```python
from build123d import *

# Parameters (mm, degrees)
SKETCH1_R            = 10
BOSS_EXTRUDE1_DEPTH  = 30
SKETCH2_R            = 12.5
BOSS_EXTRUDE5_DEPTH  = 60
SKETCH5_R            = 14
BOSS_EXTRUDE8_DEPTH  = 70
SKETCH7_R            = 16
BOSS_EXTRUDE9_DEPTH  = 76
SKETCH8_R            = 14
BOSS_EXTRUDE13_DEPTH = 24
SKETCH12_R           = 12.5
BOSS_EXTRUDE15_DEPTH = 150
SKETCH14_R           = 11.5
BOSS_EXTRUDE16_DEPTH = 70
SKETCH15_R           = 10
BOSS_EXTRUDE17_DEPTH = 20
CUT_EXTRUDE1_DEPTH   = 6
CUT_EXTRUDE2_DEPTH   = 8
SKETCH18_R           = 14
CUT_EXTRUDE3_DEPTH   = 264
SKETCH19_R           = 14
BOSS_EXTRUDE18_DEPTH = 45
SKETCH20_R           = 12.5
BOSS_EXTRUDE19_DEPTH = 139
SKETCH21_R           = 11.5
BOSS_EXTRUDE20_DEPTH = 60
SKETCH22_R           = 10
BOSS_EXTRUDE21_DEPTH = 20
CUT_EXTRUDE4_DEPTH   = 8
CUT_EXTRUDE5_DEPTH   = 8
SKETCH26_W           = 1.2
SKETCH26_H           = 1.8
SKETCH30_W           = 1.2
SKETCH30_H           = 1.8
SKETCH31_W           = 1.2
SKETCH31_H           = 1.8
SKETCH34_W           = 1.2
SKETCH34_H           = 1.8
SKETCH35_R           = 14
BOSS_EXTRUDE22_DEPTH = 56
SKETCH36_W           = 1.2
SKETCH36_H           = 1.8


with BuildPart() as part:
    # Sketch1 → Boss-Extrude1 (new body)
    with BuildSketch(Plane(origin=(0, 0, 0), x_dir=(0, 0, -1), z_dir=(1, 0, 0))):
        Circle(SKETCH1_R)
    extrude(amount=BOSS_EXTRUDE1_DEPTH)

    # Sketch2 → Boss-Extrude5 (add)
    with BuildSketch(Plane(origin=(30, 0, 0), x_dir=(0, 0, -1), z_dir=(1, 0, 0))):
        Circle(SKETCH2_R)
    extrude(amount=BOSS_EXTRUDE5_DEPTH)

    # Sketch5 → Boss-Extrude8 (add)
    with BuildSketch(Plane(origin=(90, 0, 0), x_dir=(0, 0, -1), z_dir=(1, 0, 0))):
        Circle(SKETCH5_R)
    extrude(amount=BOSS_EXTRUDE8_DEPTH)

    # Sketch7 → Boss-Extrude9 (add)
    with BuildSketch(Plane(origin=(160, 0, 0), x_dir=(0, 0, -1), z_dir=(1, 0, 0))):
        Circle(SKETCH7_R)
    extrude(amount=BOSS_EXTRUDE9_DEPTH)

    # Sketch8 → Boss-Extrude13 (add)
    with BuildSketch(Plane(origin=(236, 0, 0), x_dir=(0, 0, -1), z_dir=(1, 0, 0))):
        Circle(SKETCH8_R)
    extrude(amount=BOSS_EXTRUDE13_DEPTH)

    # Sketch12 → Boss-Extrude15 (add)
    with BuildSketch(Plane(origin=(260, 0, 0), x_dir=(0, 0, -1), z_dir=(1, 0, 0))):
        Circle(SKETCH12_R)
    extrude(amount=BOSS_EXTRUDE15_DEPTH)

    # Sketch14 → Boss-Extrude16 (add)
    with BuildSketch(Plane(origin=(410, 0, 0), x_dir=(0, 0, -1), z_dir=(1, 0, 0))):
        Circle(SKETCH14_R)
    extrude(amount=BOSS_EXTRUDE16_DEPTH)

    # Sketch15 → Boss-Extrude17 (add)
    with BuildSketch(Plane(origin=(480, 0, 0), x_dir=(0, 0, -1), z_dir=(1, 0, 0))):
        Circle(SKETCH15_R)
    extrude(amount=BOSS_EXTRUDE17_DEPTH)

    # Sketch16 → Cut-Extrude1 (cut)
    with BuildSketch(Plane.XY.offset(10)):
        with BuildLine():
            Line((5, 4), (25, 4))
            ThreePointArc((25, 4), (29, 0), (25, -4))
            Line((25, -4), (5, -4))
            ThreePointArc((5, -4), (1, 0), (5, 4))
        make_face()
    extrude(amount=-CUT_EXTRUDE1_DEPTH, mode=Mode.SUBTRACT)

    # Sketch17 → Cut-Extrude2 (cut)
    with BuildSketch(Plane.XY.offset(14)):
        with BuildLine():
            Line((125, 5), (153, 5))
            ThreePointArc((153, 5), (158, 0), (153, -5))
            Line((153, -5), (125, -5))
            ThreePointArc((125, -5), (120, 0), (125, 5))
        make_face()
    extrude(amount=-CUT_EXTRUDE2_DEPTH, mode=Mode.SUBTRACT)

    # Sketch18 → Cut-Extrude3 (cut)
    with BuildSketch(Plane(origin=(236, 0, 0), x_dir=(0, 0, -1), z_dir=(1, 0, 0))):
        Circle(SKETCH18_R)
    extrude(amount=CUT_EXTRUDE3_DEPTH, mode=Mode.SUBTRACT)

    # Sketch19 → Boss-Extrude18 (add)
    with BuildSketch(Plane(origin=(236, 0, 0), x_dir=(0, 0, -1), z_dir=(1, 0, 0))):
        Circle(SKETCH19_R)
    extrude(amount=BOSS_EXTRUDE18_DEPTH)

    # Sketch20 → Boss-Extrude19 (add)
    with BuildSketch(Plane(origin=(281, 0, 0), x_dir=(0, 0, -1), z_dir=(1, 0, 0))):
        Circle(SKETCH20_R)
    extrude(amount=BOSS_EXTRUDE19_DEPTH)

    # Sketch21 → Boss-Extrude20 (add)
    with BuildSketch(Plane(origin=(420, 0, 0), x_dir=(0, 0, -1), z_dir=(1, 0, 0))):
        Circle(SKETCH21_R)
    extrude(amount=BOSS_EXTRUDE20_DEPTH)

    # Sketch22 → Boss-Extrude21 (add)
    with BuildSketch(Plane(origin=(480, 0, 0), x_dir=(0, 0, -1), z_dir=(1, 0, 0))):
        Circle(SKETCH22_R)
    extrude(amount=BOSS_EXTRUDE21_DEPTH)

    # Sketch24 → Cut-Extrude4 (cut)
    with BuildSketch(Plane.XY.offset(14)):
        with BuildLine():
            Line((244.5, 6), (272.5, 6))
            ThreePointArc((272.5, 6), (278.5, 0), (272.5, -6))
            Line((272.5, -6), (244.5, -6))
            ThreePointArc((244.5, -6), (238.5, 0), (244.5, 6))
        make_face()
    extrude(amount=-CUT_EXTRUDE4_DEPTH, mode=Mode.SUBTRACT)

    # Sketch25 → Cut-Extrude5 (cut)
    with BuildSketch(Plane.XY.offset(11.5)):
        with BuildLine():
            Line((428.5, 6), (451.5, 6))
            ThreePointArc((451.5, 6), (457.5, 0), (451.5, -6))
            Line((451.5, -6), (428.5, -6))
            ThreePointArc((428.5, -6), (422.5, 0), (428.5, 6))
        make_face()
    extrude(amount=-CUT_EXTRUDE5_DEPTH, mode=Mode.SUBTRACT)

    # Sketch26 → Cut-Revolve2 (revolve, cut)
    with BuildSketch(Plane(origin=(0, 0, 0), x_dir=(1, 0, 0), z_dir=(0, 1, 0))):
        with Locations((71.13362974, -11.6)):
            Rectangle(SKETCH26_W, SKETCH26_H)
    revolve(axis=Axis((30.471957332, 0, 0), (1, 0, 0)), mode=Mode.SUBTRACT)

    # Sketch30 → Cut-Revolve5 (revolve, cut)
    with BuildSketch(Plane(origin=(0, 0, 0), x_dir=(1, 0, 0), z_dir=(0, 1, 0))):
        with Locations((462.1, -10.6)):
            Rectangle(SKETCH30_W, SKETCH30_H)
    revolve(axis=Axis((419.735953091, 0, 0), (1, 0, 0)), mode=Mode.SUBTRACT)

    # Sketch31 → Cut-Revolve6 (revolve, cut)
    with BuildSketch(Plane(origin=(0, 0, 0), x_dir=(1, 0, 0), z_dir=(0, 1, 0))):
        with Locations((400.6, -11.6)):
            Rectangle(SKETCH31_W, SKETCH31_H)
    revolve(axis=Axis((419.735953091, 0, 0), (-1, 0, 0)), mode=Mode.SUBTRACT)

    # Sketch34 → Cut-Revolve8 (revolve, cut)
    with BuildSketch(Plane(origin=(0, 0, 0), x_dir=(1, 0, 0), z_dir=(0, 1, 0))):
        with Locations((115.4, -13.1)):
            Rectangle(SKETCH34_W, SKETCH34_H)
    revolve(axis=Axis((91.001068782, 0, 0), (1, 0, 0)), mode=Mode.SUBTRACT)

    # Sketch35 → Boss-Extrude22 (add)
    with BuildSketch(Plane(origin=(281, 0, 0), x_dir=(0, 0, -1), z_dir=(1, 0, 0))):
        with Locations(Location((0, 0, 0), (0, 0, 180))):
            Circle(SKETCH35_R)
    extrude(amount=BOSS_EXTRUDE22_DEPTH)

    # Sketch36 → Cut-Revolve9 (revolve, cut)
    with BuildSketch(Plane(origin=(0, 0, 0), x_dir=(1, 0, 0), z_dir=(0, 1, 0))):
        with Locations((283.1, -13.1)):
            Rectangle(SKETCH36_W, SKETCH36_H)
    revolve(axis=Axis((235.166197804, 0, 0), (1, 0, 0)), mode=Mode.SUBTRACT)


solid = part.part
```
CAD build for the part. Positions are in the model's coordinates, mm. A direction names the side the tool comes from. Round coordinates to 2 decimals unless told otherwise and drop trailing zeros. Order: outer loops, then holes, each group sorted by start corner. A loop starts at its lowest first (then second) coordinate and runs counter-clockwise, first axis right, second up.
Item 1: Probe line 1 along X through (y, z) = (9, -7); line 2 along X through (y, z) = (8.5, -9); line 3 along X through (y, z) = (-9.5, 7). List the from-to ranges inside material, lowest first.
Item 2: Pin check, flat tips, straight feed: pin 1 (5 mm diameter, centred on x = 449.5, z = 5, fed in from +Y) (3 decimals); pin 2 (6 mm diameter, centred on y = -7.5, z = -11, fed in from +X); pin 3 (2.5 mm diameter, centred on x = 19, z = 6, fed in from +Y). Stop position of each tip, or through.
Item 3: Saw through at B-B on x = 316. Write the cut outline in (y, z).
Item 4: Mould opens along Y. For faces 4 (the face through (457.5, 0.1, 7.6)), 5 (the face through (440, 0, 3.5)), 6 (the face through (70.534, -9.3, -5.6)), 7 (the face through (462.108, -2.914, 9.252)) say: pulls with the +Y half, pulls with the -Y half, needs draft (parallel to the pull), parting line crosses it, or undercut.
Item 5: Tool access for faces 1 (the face through (238.5, -0.1, 10.1)), 2 (the face through (461.5, 8, -6)), 3 (the face through (236, -14.15, 0.07)): list every direction of +Z, -Z, +X, -X, +Y, -Y with a clear straight run to the whole face (end or side of a thin tool).
Item 6: Saw through at A-A on x = 382. Write the cut outline in (y, z).
Item 7: Saw through at C-C on x = 143. Write the cut outline in (y, z).
Reported:
1. line 1: x = 30 to 70.53, 71.73 to 400, 401.2 to 461.5, 462.7 to 480
1. line 2: x = 30 to 70.53, 71.73 to 114.8, 116 to 282.5, 283.7 to 400, 401.2 to 420
1. line 3: x = 30 to 70.53, 71.73 to 400, 401.2 to 420
2. pin 1: stops at y = 11.225
2. pin 2: stops at x = 480
2. pin 3: stops at y = 8.8
3. outline: circle Ø28 at (0, 0)
4. face 4: undercut
4. face 5: undercut
4. face 6: needs draft
4. face 7: parting line crosses it
5. face 1: +Z
5. face 2: none
5. face 3: +X
6. outline: circle Ø25 at (0, 0)
7. outline: (-5, 6) - (-5, 13.08) arc R14 ccw (long way) to (5, 13.08) - (5, 6) - close
